Verification items for the finished model (mm, model axes). Round coordinates to 2 decimals unless told otherwise and drop trailing zeros. Loops run counter-clockwise (first coordinate to the right, second up) from the corner with the lowest first, then second, coordinate; pieces in that order, holes last. Notation, with made-up numbers: (62.25, 23.25) -> (91.25, 23.25) arc R4 cw to (91.25, 29.25) -> close; hole circle Ø6 at (-1, 16). An arc over 180 degrees is marked (long way). Write item = value, one per line.
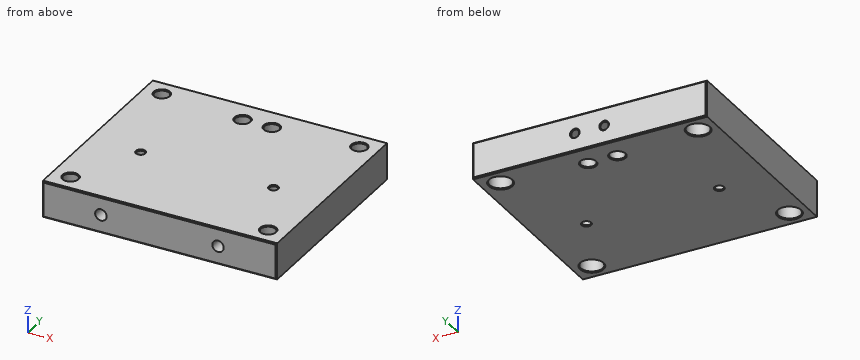
```python
from build123d import *

# Parameters (mm, degrees)
SKETCH1_W                       = 101.6
SKETCH1_H                       = 88.9
BOSS_EXTRUDE1_DEPTH             = 15.875
F_8_32_TAPPED_HOLE1_D           = 3.4544
F_8_32_TAPPED_HOLE1_DEPTH       = 9.652
F_8_32_TAPPED_HOLE1_CSINK_D     = 4.1656
F_8_32_TAPPED_HOLE1_CSINK_ANGLE = 90
F_8_32_TAPPED_HOLE1_TIP         = 1.037806461
F_1_4_0_25_DIAMETER_HOLE1_D     = 6.35
F_1_4_0_25_DIAMETER_HOLE1_DEPTH = 25.4
F_1_4_0_25_DIAMETER_HOLE1_TIP   = 1.907732465
F_8_32_TAPPED_HOLE2_D           = 3.4544
F_9_0_196_DIAMETER_HOLE1_D      = 4.9784
F_9_0_196_DIAMETER_HOLE1_DEPTH  = 12.7
F_9_0_196_DIAMETER_HOLE1_TIP    = 1.495662253
HOLE1_D                         = 6.35
HOLE1_DEPTH                     = 15.875
HOLE1_CBORE_D                   = 9.525
HOLE1_CBORE_DEPTH               = 9.525
HOLE1_TIP                       = 1.907732465
CHAMFER1_SIZE                   = 0.508
CHAMFER2_SIZE                   = 0.381


with BuildPart() as part:
    # Sketch1 → Boss-Extrude1 (new body)
    with BuildSketch(Plane.XY):
        with Locations((-50.8, 44.45)):
            Rectangle(SKETCH1_W, SKETCH1_H)
    extrude(amount=BOSS_EXTRUDE1_DEPTH)

    # #8-32 Tapped Hole1
    with Locations(Plane(origin=(0, 88.9, 0), x_dir=(1, 0, 0), z_dir=(0, 1, 0))):
        with Locations((-44.45, -7.9375), (-57.15, -7.9375)):
            CounterSinkHole(F_8_32_TAPPED_HOLE1_D / 2, F_8_32_TAPPED_HOLE1_CSINK_D / 2, depth=F_8_32_TAPPED_HOLE1_DEPTH, counter_sink_angle=F_8_32_TAPPED_HOLE1_CSINK_ANGLE)
            with Locations((0, 0, -(F_8_32_TAPPED_HOLE1_DEPTH + F_8_32_TAPPED_HOLE1_TIP / 2))):  # 118° drill point
                Cone(0, F_8_32_TAPPED_HOLE1_D / 2, F_8_32_TAPPED_HOLE1_TIP, mode=Mode.SUBTRACT)

    # 1/4 (0.25) Diameter Hole1
    with Locations(Plane.XY.offset(15.875)):
        with Locations((-44.45, 78.210193539), (-57.15, 78.210193539)):
            Hole(F_1_4_0_25_DIAMETER_HOLE1_D / 2, depth=F_1_4_0_25_DIAMETER_HOLE1_DEPTH)
            with Locations((0, 0, -(F_1_4_0_25_DIAMETER_HOLE1_DEPTH + F_1_4_0_25_DIAMETER_HOLE1_TIP / 2))):  # 118° drill point
                Cone(0, F_1_4_0_25_DIAMETER_HOLE1_D / 2, F_1_4_0_25_DIAMETER_HOLE1_TIP, mode=Mode.SUBTRACT)

    # #8-32 Tapped Hole2 (through all)
    with Locations(Plane(origin=(0, 0, 0), x_dir=(-1, 0, 0), z_dir=(0, 0, -1))):
        with Locations((21.675, 37.592), (79.3203, 37.592)):
            Hole(F_8_32_TAPPED_HOLE2_D / 2)

    # #9 (0.196) Diameter Hole1
    with Locations(Plane(origin=(0, 0, 0), x_dir=(-1, 0, 0), z_dir=(0, -1, 0))):
        with Locations((76.2, -7.9375), (25.4, -7.9375)):
            Hole(F_9_0_196_DIAMETER_HOLE1_D / 2, depth=F_9_0_196_DIAMETER_HOLE1_DEPTH)
            with Locations((0, 0, -(F_9_0_196_DIAMETER_HOLE1_DEPTH + F_9_0_196_DIAMETER_HOLE1_TIP / 2))):  # 118° drill point
                Cone(0, F_9_0_196_DIAMETER_HOLE1_D / 2, F_9_0_196_DIAMETER_HOLE1_TIP, mode=Mode.SUBTRACT)

    # Hole1
    with Locations(Plane(origin=(0, 0, 0), x_dir=(1, 0, 0), z_dir=(0, 0, -1))):
        with Locations((-7.9375, -7.9375), (-93.6625, -80.9625), (-93.6625, -7.9375), (-7.9375, -80.9625)):
            CounterBoreHole(HOLE1_D / 2, HOLE1_CBORE_D / 2, HOLE1_CBORE_DEPTH, depth=HOLE1_DEPTH)
            with Locations((0, 0, -(HOLE1_DEPTH + HOLE1_TIP / 2))):  # 118° drill point
                Cone(0, HOLE1_D / 2, HOLE1_TIP, mode=Mode.SUBTRACT)

    # Chamfer1
    chamfer1_edges = [part.edges().sort_by_distance(p)[0] for p in [
        (-50.8, 0, 15.875),
        (-50.8, 0, 0),
        (-50.8, 88.9, 0),
        (-50.8, 88.9, 15.875),
        (0, 0, 7.9375),
        (-101.6, 0, 7.9375),
        (-101.6, 88.9, 7.9375),
        (0, 88.9, 7.9375),
    ]]
    chamfer(chamfer1_edges, length=CHAMFER1_SIZE)

    # Chamfer2
    chamfer2_edges = [part.edges().sort_by_distance(p)[0] for p in [
        (-53.975, 78.210193539, 0),
        (-53.975, 78.210193539, 15.875),
        (-41.275, 78.210193539, 0),
        (-41.275, 78.210193539, 15.875),
        (-23.4022, 37.592, 0),
        (-23.4022, 37.592, 15.875),
        (-81.0475, 37.592, 0),
        (-81.0475, 37.592, 15.875),
        (-12.7, 80.9625, 0),
        (-4.7625, 80.9625, 15.875),
        (-98.425, 7.9375, 0),
        (-90.4875, 7.9375, 15.875),
        (-98.425, 80.9625, 0),
        (-90.4875, 80.9625, 15.875),
        (-12.7, 7.9375, 0),
        (-4.7625, 7.9375, 15.875),
    ]]
    chamfer(chamfer2_edges, length=CHAMFER2_SIZE)


solid = part.part
```
(1) Material ranges on probe 1 along Y at (x, z) = (-9, 2); probe 2 along Z at (x, y) = (-76.2, 9.25) (3 decimals); probe 3 along X at (y, z) = (75.5, 3.25), recorded low to high. Write a range as from..to.
Filled sheet:
probe_1 = 0..3.3, 12.58..76.32, 85.6..88.9
probe_2 = 0..5.448, 10.427..15.875
probe_3 = -101.6..-58.8, -55.5..-46.1, -42.8..0
(2) Sectioned sample at A-A, the plane x = -57.15. Record the cut outline in (y, z) (3 decimals), and give its area (3 significant figures).
Filled sheet:
outline = (0, 0.508) -> (0.508, 0) -> (74.654, 0) -> (75.035, 0.381) -> (75.035, 15.494) -> (74.654, 15.875) -> (0.508, 15.875) -> (0, 15.367) -> close; (81.385, 0.381) -> (81.766, 0) -> (88.392, 0) -> (88.9, 0.508) -> (88.9, 5.855) -> (88.544, 6.21) -> (81.385, 6.21) -> close; (81.385, 9.665) -> (88.544, 9.665) -> (88.9, 10.02) -> (88.9, 15.367) -> (88.392, 15.875) -> (81.766, 15.875) -> (81.385, 15.494) -> close
area = 1,280 mm2
(3) Sectioned sample at B-B, the plane z = 3.25. Count the separate pieces of the cut face and the enclosed holes in it, and give its area (3 significant figures).
Filled sheet:
separate_pieces = 1
enclosed_holes = 8
area = 8,660 mm2
(4) Go/stop test with a flat-tipped pin: pin 1 Ø4 at (x, z) = (-25.4, 7.94) entering from -Y. Record where the tip stops, or that it passes through.
Filled sheet:
pin_1 = 12.99
